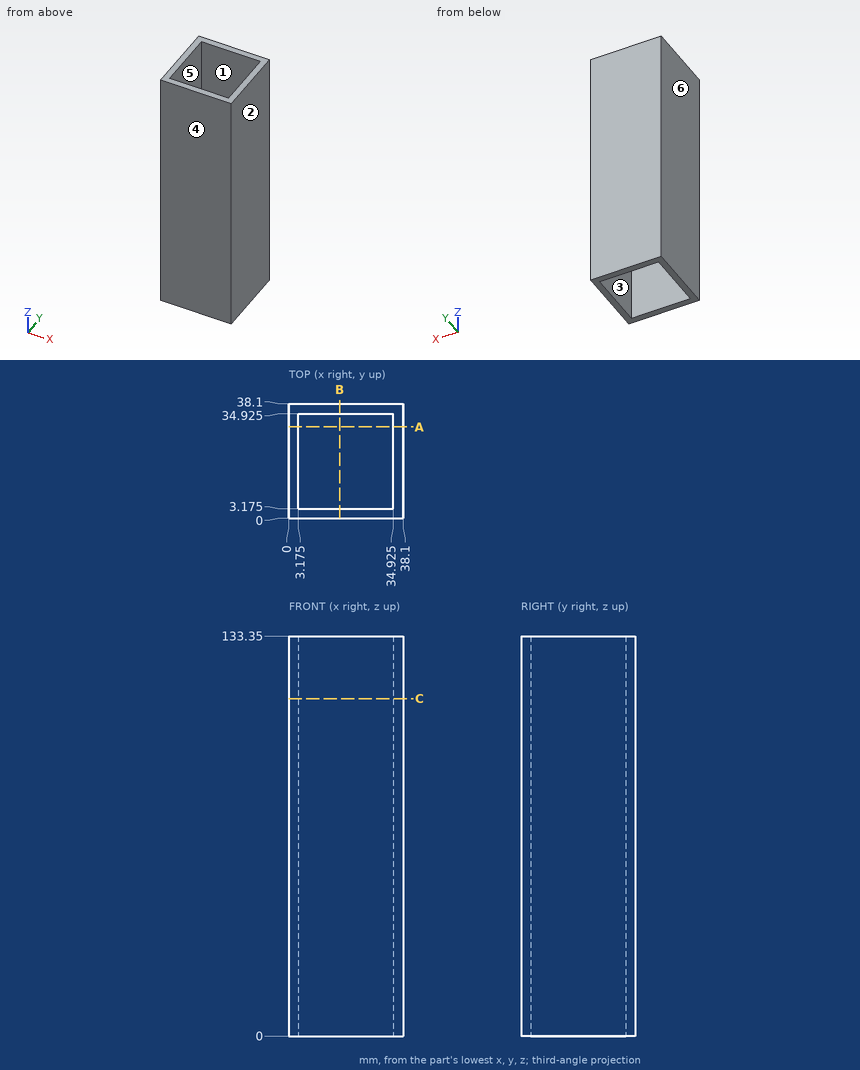
Can you work these out from the drawing? Everything is in mm from the part's minimum corner. A direction names the side the tool comes from. Coordinates: 2 decimals unless noted, no trailing zeros. Loops run counter-clockwise (first coordinate to the right, second up) from the corner with the lowest first, then second, coordinate; pieces in that order, holes last. Notation, with made-up numbers: (78, 41.5) - (113, 41.5) arc R29 ccw to (113, 65.5) - close; hole circle Ø4 at (-13, -40). An arc over 180 degrees is marked (long way). Use a Markdown table: item, result.
Item 1: I want a section at A-A on y = 30.5. Please give me the cut outline in (x, z) (3 decimals), and give its area (3 significant figures).
Numbers:
| item | result |
|---|---|
| outline | (0, 0) - (3.175, 0) - (3.175, 133.35) - (0, 133.35) - close; (34.925, 0) - (38.1, 0) - (38.1, 133.35) - (34.925, 133.35) - close |
| area | 847 mm2 |
Item 2: I want a section at C-C on z = 112.5. Please give me the cut outline in (x, y) (3 decimals), and give its area (3 significant figures).
Numbers:
| item | result |
|---|---|
| outline | (0, 0) - (38.1, 0) - (38.1, 38.1) - (0, 38.1) - close; hole (3.175, 3.175) - (34.925, 3.175) - (34.925, 34.925) - (3.175, 34.925) - close |
| area | 444 mm2 |
Item 3: For the marked faces 1 and 2, which set-ups out of +Z, -Z, +X, -X, +Y, -Y let a thin tool reach every point of the face, with its end or its side?
Numbers:
| item | result |
|---|---|
| face 1 | +Z, -Z |
| face 2 | +Z, -Z, +X, +Y, -Y |
Item 4: We'd pull the mould along X, two halves only. Please class the marked faces 3, 4, 5 and 6: released by +X, released by -X, zero draft, split by the parting line, or undercut.
Numbers:
| item | result |
|---|---|
| face 3 | undercut |
| face 4 | zero draft |
| face 5 | undercut |
| face 6 | released by -X |
Item 5: If I drill on probe 1 along X at (y, z) = (4.5, 110) (3 decimals), over which ranges is the centre line in solid material (lowest first)? Write a range as from..to.
Numbers:
| item | result |
|---|---|
| probe 1 | x = 0..3.175, 34.925..38.1 |
